```python
from build123d import *

# Parameters (mm, degrees)
SKETCH2_W           = 127
SKETCH2_H           = 57.404
SKETCH2_R           = 4.864
BOSS_EXTRUDE1_DEPTH = 1.5875


with BuildPart() as part:
    # Sketch2 → Boss-Extrude1 (new body)
    with BuildSketch(Plane.XY):
        with Locations((63.5, 28.702)):
            Rectangle(SKETCH2_W, SKETCH2_H)
        with Locations((63.5, 12.500102)):
            Circle(SKETCH2_R, mode=Mode.SUBTRACT)
    extrude(amount=-BOSS_EXTRUDE1_DEPTH)

    # Sketch3 → 1/4 NPT Tapped Hole1 (revolve, cut)
    with BuildSketch(Plane(origin=(19.05, 16.129, 0), x_dir=(0, -1, 0), z_dir=(1, 0, 0))):
        Polygon((0, 0), (0, 1.5875), (5.5626, 1.5875), (5.5626, 9.906), (6.557984794, 9.906), (6.8545837, 0), align=None)
    revolve(axis=Axis((19.05, 16.129, 6.35), (0, 0, -1)), mode=Mode.SUBTRACT)


solid = part.part
```
Here's how the part is built. I have some questions about the finished solid (model axes, mm). Coordinates: 2 decimals unless noted, no trailing zeros. Loops run counter-clockwise (first coordinate to the right, second up) from the corner with the lowest first, then second, coordinate; pieces in that order, holes last. Notation, with made-up numbers: (-12, 87) - (29, 87) arc R19 ccw to (29, 102) - close; hole circle Ø9 at (27, -15). An arc over 180 degrees is marked (long way). Answer as CSV lines item,"result".
Q1. If we section it at C-C, the plane x = 19.05: Write out the boundary of the cut face in (y, z).
Response:
outline,"(0, -1.59) - (9.32, -1.59) - (9.27, 0) - (0, 0) - close; (22.94, -1.59) - (57.4, -1.59) - (57.4, 0) - (22.98, 0) - close"
Q2. If we section it at D-D, the plane y = 15: Give the number of separate pieces and of enclosed holes in the cut face, and give its area (3 significant figures).
Response:
separate pieces,"3"
enclosed holes,"0"
area,"167 mm2"
Q3. We'd pull the mould along X, two halves only. Please class faces 1 (the face through (58.64, 12.71, -0.78)), 2 (the face through (63, 29, 0)), 3 (the face through (25.106, 12.979, -0.959)): pulls with the +X half, pulls with the -X half, needs draft (parallel to the pull), parting line crosses it, or undercut.
Response:
face 1,"undercut"
face 2,"needs draft"
face 3,"undercut"
Q4. If I drill on L1, parallel to Y at x = 63.5, z = -0.45; L2, parallel to X at y = 12.5, z = -0.95; L3, parallel to Y at x = 59.5, z = -0.8, over which ranges is the centre line in solid material (lowest first)? Write a range as [from, to].
Response:
L1,"[0, 7.64], [17.36, 57.4]"
L2,"[0, 13.27], [24.83, 58.64], [68.36, 127]"
L3,"[0, 9.73], [15.27, 57.4]"
Q5. If we section it at A-A, the plane x = 63.5: Write out the boundary of the cut face in (y, z), and give its area (3 significant figures).
Response:
outline,"(0, -1.59) - (7.64, -1.59) - (7.64, 0) - (0, 0) - close; (17.36, -1.59) - (57.4, -1.59) - (57.4, 0) - (17.36, 0) - close"
area,"75.7 mm2"
Q6. If we section it at B-B, the plane z = -1: Write out the boundary of the cut face in (x, y), and give its area (3 significant figures).
Response:
outline,"(0, 0) - (127, 0) - (127, 57.4) - (0, 57.4) - close; hole circle Ø13.65 at (19.05, 16.13); hole circle Ø9.73 at (63.5, 12.5)"
area,"7,070 mm2"
